```python
from build123d import *

# Parameters (mm, degrees)
ESQUISSE1_R        = 2
BOSS_EXTRU_1_DEPTH = 15
BOSS_EXTRU_2_DEPTH = 10


with BuildPart() as part:
    # Esquisse1 → Boss.-Extru.1 (new, symmetric)
    with BuildSketch(Plane(origin=(0, 0, 0), x_dir=(0, 0, -1), z_dir=(1, 0, 0))):
        Circle(ESQUISSE1_R)
    extrude(amount=BOSS_EXTRU_1_DEPTH, both=True)

    # Esquisse1_4 → Boss.-Extru.2 (add, symmetric)
    with BuildSketch(Plane(origin=(0, 0, 0), x_dir=(0, 0, -1), z_dir=(1, 0, 0))):
        Polygon((-2.31, 4.001037365), (2.31, 4.001037365), (4.62, 0), (2.31, -4.001037365), (-2.31, -4.001037365), (-4.62, 0), align=None)
    extrude(amount=BOSS_EXTRU_2_DEPTH, both=True)


solid = part.part
```
Part model, mm, in its own coordinate system. A direction names the side the tool comes from. Give positions to 0.01 mm unless a question says otherwise; leave off trailing zeros. Write each loop counter-clockwise with the first axis right and the second up, starting at its lowest first coordinate (ties: lowest second). Pieces come first, ordered by that corner, then holes. Notation, with made-up numbers: (36, -18.5) -> (41, -18.5) arc R18 ccw to (41, -14.5) -> close; hole circle Ø6 at (47.25, 61.5). An arc over 180 degrees is marked (long way). Put each result on its own line as item: value. Start each with the question number.
Item 1: Cut at B-B (x = -2.75). List the corners of the cut face in (y, z).
Item 2: Cut at D-D (x = 10.75). List the corners of the cut face in (y, z), then the cut area to 3 significant figures.
Item 3: Cut at C-C (y = -2.5). List the corners of the cut face in (x, z), then the cut area to 3 significant figures.
Item 4: Cut at A-A (z = 0). List the corners of the cut face in (x, y).
Item 5: Pin check, flat tip, straight feed: pin 1 Ø1 at (x, y) = (9, 3) entering from +Z. Stop position of the tip, or through.
Item 6: Which spindle directions (+Z, -Z, +X, -X, +Y, -Y) get a long thin tool onto all of the face, cutting with end or side? Do faces 1 (the face through (-10, 2, 1)), 2 (the face through (0.14, 2.03, -3.45)), 3 (the face through (10, 2, 1)). Say none if no direction does.
Item 7: Wall check: L1, parallel to X at y = 1, z = -3.25; L2, parallel to Z at x = 0.75, y = 0.25; L3, parallel to Z at x = 9.75, y = -2. Give the ranges that are in metal, low to high. Write a range as [from, to].
Answer list:
1. outline: (-4, -2.31) -> (0, -4.62) -> (4, -2.31) -> (4, 2.31) -> (0, 4.62) -> (-4, 2.31) -> close
2. outline: circle Ø4 at (0, 0)
2. area: 12.6 mm2
3. outline: (-10, -3.18) -> (10, -3.18) -> (10, 3.18) -> (-10, 3.18) -> close
3. area: 127 mm2
4. outline: (-15, -2) -> (-10, -2) -> (-10, -4) -> (10, -4) -> (10, -2) -> (15, -2) -> (15, 2) -> (10, 2) -> (10, 4) -> (-10, 4) -> (-10, 2) -> (-15, 2) -> close
5. pin 1: stops at z = 3.18
6. face 1: -X
6. face 2: -Z, +X, -X, +Y
6. face 3: +X
7. L1: x = [-10, 10]
7. L2: z = [-4.48, 4.48]
7. L3: z = [-3.47, 3.47]
